Part model, mm, in its own coordinate system. Face numbers are marked on the shaded views. A direction names the side the tool comes from. Coordinates: 2 decimals unless noted, no trailing zeros. Loops run counter-clockwise (first coordinate to the right, second up) from the corner with the lowest first, then second, coordinate; pieces in that order, holes last. Notation, with made-up numbers: (24.5, 21) - (53.5, 21) arc R34 ccw to (53.5, 57) - close; hole circle Ø4 at (74, 33). An arc over 180 degrees is marked (long way). Use a Markdown table: item, result. Add a question column.
1. Drop flat-ended pins along their axis: pin 1 (4 mm diameter, centred on y = 13, z = -15.5, fed in from -X); pin 2 (3 mm diameter, centred on y = -15, z = -8, fed in from -X); pin 3 (23.5 mm diameter, centred on x = -1200, z = 0, fed in from +Y). Give the stop position or say it passes through.
2. Band-saw the part on A-A, the plane z = 0. Give the cut face in (x, y).
3. Wall check: probe 1 along Z at (x, y) = (-1102, 0); probe 2 along Z at (x, y) = (-1200, -14); probe 3 along Y at (x, z) = (-1159.5, -4.5). Give the ranges that are in metal, low to high. Write a range as [from, to].
4. Pull direction X, two halves, no side cores. Call the marked faces 6, 7, 8 and 9: pulls with the +X half, pulls with the -X half, needs draft (parallel to the pull), parting line crosses it, or undercut.
5. Band-saw the part on B-B, the plane x = -1132. Give the cut face in (y, z).
6. Band-saw the part on C-C, the plane y = 19.5. Give the cut face in (x, z), plus the area to 3 significant figures.
7. Band-saw the part on D-D, the plane x = -1105.5. Give the cut face in (y, z), plus the area to 3 significant figures.
8. 3-axis set-ups, long thin cutter, end or side, ignore diameter. For the marked faces 1, 2, 3, 4 and 5: which of +Z, -Z, +X, -X, +Y, -Y reach the whole face in a straight line?
from build123d import *

# Parameters (mm, degrees)
SKETCH007_R      = 13
EXTRUDE_DEPTH    = 65
SKETCH017_R      = 12
EXTRUDE008_DEPTH = 40
EXTRUDE007_DEPTH = 75
PAD_DEPTH        = 25


with BuildPart() as extrude_body:
    # Sketch007 (on Face6 of Pad) → Extrude (new body)
    with BuildSketch(Plane.XZ.offset(25)):
        Circle(SKETCH007_R)
    extrude(amount=-EXTRUDE_DEPTH)


with BuildPart() as extrude008:
    # Sketch017 → Extrude008 (new body)
    with BuildSketch(Plane.YZ.offset(90)):
        Circle(SKETCH017_R)
    extrude(amount=EXTRUDE008_DEPTH)


with BuildPart() as extrude007:
    # Sketch016 → Extrude007 (new body, symmetric)
    with BuildSketch(Plane.XY):
        with BuildLine():
            Line((-30, 11.5), (26, 11.5))
            Line((26, 11.5), (26, 14))
            ThreePointArc((28, 16), (26.585786, 15.414214), (26, 14))
            Line((28, 16), (73, 16))
            ThreePointArc((75, 14), (74.414214, 15.414214), (73, 16))
            Line((75, 14), (75, -14))
            ThreePointArc((73, -16), (74.414214, -15.414214), (75, -14))
            Line((73, -16), (28, -16))
            ThreePointArc((26, -14), (26.585786, -15.414214), (28, -16))
            Line((26, -14), (26, -11.5))
            Line((26, -11.5), (-30, -11.5))
            Line((-30, -11.5), (-30, 11.5))
        make_face()
    extrude(amount=EXTRUDE007_DEPTH, both=True)


with BuildPart() as obj1:
    # Sketch → Pad (new body, symmetric)
    with BuildSketch(Plane.XZ):
        with BuildLine():
            Line((115, 30), (0, 30))
            ThreePointArc((0, 30), (-30, 0), (0, -30))
            Line((0, -30), (115, -30))
            Line((115, -30), (115, 30))
        make_face()
    extrude(amount=PAD_DEPTH, both=True)

    # Cut: cut Extrude007
    add(extrude007.part, mode=Mode.SUBTRACT)

    # Cut007: cut Extrude008
    add(extrude008.part, mode=Mode.SUBTRACT)

    # Cut008: cut Extrude body
    add(extrude_body.part, mode=Mode.SUBTRACT)


with BuildPart() as obj1_1:
    # Cut008 placement: moved
    add(obj1.part.moved(Location((-1200, 0, 0))))


solid = obj1_1.part
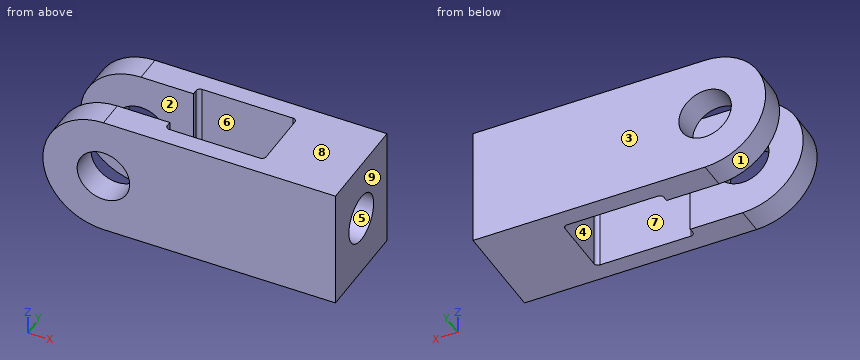
Geometry check:
| question | item | result |
|---|---|---|
| 1 | pin 1 | stops at x = -1226.79 |
| 1 | pin 2 | stops at x = -1229.29 |
| 1 | pin 3 | passes through |
| 2 | outline | (-1230, -25) - (-1213, -25) - (-1213, -11.5) - (-1230, -11.5) - close; (-1230, 11.5) - (-1213, 11.5) - (-1213, 25) - (-1230, 25) - close; (-1187, -25) - (-1085, -25) - (-1085, -12) - (-1110, -12) - (-1110, 12) - (-1085, 12) - (-1085, 25) - (-1187, 25) - (-1187, 11.5) - (-1174, 11.5) - (-1174, 14) arc R2 cw to (-1172, 16) - (-1127, 16) arc R2 cw to (-1125, 14) - (-1125, -14) arc R2 cw to (-1127, -16) - (-1172, -16) arc R2 cw to (-1174, -14) - (-1174, -11.5) - (-1187, -11.5) - close |
| 3 | probe 1 | z = [-30, -12], [12, 30] |
| 3 | probe 2 | z = [-30, -13], [13, 30] |
| 3 | probe 3 | y = [-25, -16], [16, 25] |
| 4 | face 6 | undercut |
| 4 | face 7 | undercut |
| 4 | face 8 | needs draft |
| 4 | face 9 | pulls with the +X half |
| 5 | outline | (-25, -30) - (-16, -30) - (-16, 30) - (-25, 30) - close; (16, -30) - (25, -30) - (25, 30) - (16, 30) - close |
| 6 | outline | (-1200, -30) - (-1085, -30) - (-1085, 30) - (-1200, 30) arc R30 ccw to start; hole circle Ø26 at (-1200, 0) |
| 6 | area | 7,780 mm^2 |
| 7 | outline | (-25, -30) - (25, -30) - (25, 30) - (-25, 30) - close; hole circle Ø24 at (0, 0) |
| 7 | area | 2,550 mm^2 |
| 8 | face 1 | -X, +Y, -Y |
| 8 | face 2 | +Z, -Z, -X |
| 8 | face 3 | +Z, -Z, +X, -X, +Y |
| 8 | face 4 | +Z, -Z |
| 8 | face 5 | +X |
